Answer from the drawing. Dimensions are ordinates in mm from the lowest x, y and z of the part. A direction names the side the tool comes from. Give positions to 0.01 mm unless a question says otherwise; leave off trailing zeros. Loops run counter-clockwise (first coordinate to the right, second up) from the corner with the lowest first, then second, coordinate; pieces in that order, holes last.
Item 1: Consider line 1 along Z through (x, y) = (26, 83); line 2 along Y through (x, z) = (78.5, 28.5) (1 decimal); line 3 along Z through (x, y) = (77.5, 103). Determine where each line is inside the solid, lowest interval first.
Item 2: Section D-D, the plane x = 97 is taken. Give the vertices of the cut face in (y, z) (1 decimal).
Item 3: Section B-B, the plane y = 120 is taken. Give the vertices of the cut face in (x, z).
Item 4: A tool of negligible diameter and unlimited length cuts with its end or side. For the marked faces 1 and 2, from which of +Z, -Z, +X, -X, +Y, -Y can it reach the whole face along a straight path? Write none if from no direction.
Item 5: Section A-A, the plane x = 58.5 is taken. Give the vertices of the cut face in (y, z), and give its area (3 significant figures).
Item 6: Each of these flat-tipped pins is pushed along its axis until it touches: pin 1 Ø5 at (x, y) = (98, 26.5) entering from -Z; pin 2 Ø4 at (x, y) = (122, 122.5) entering from +Z; pin 3 Ø1.5 at (x, z) = (80.5, 45.5) entering from -Y. Where does it stop, or does it pass through?
Item 7: Section C-C, the plane z = 60.5 is taken. Give the vertices of the cut face in (x, y) (1 decimal), and give its area (3 significant figures).
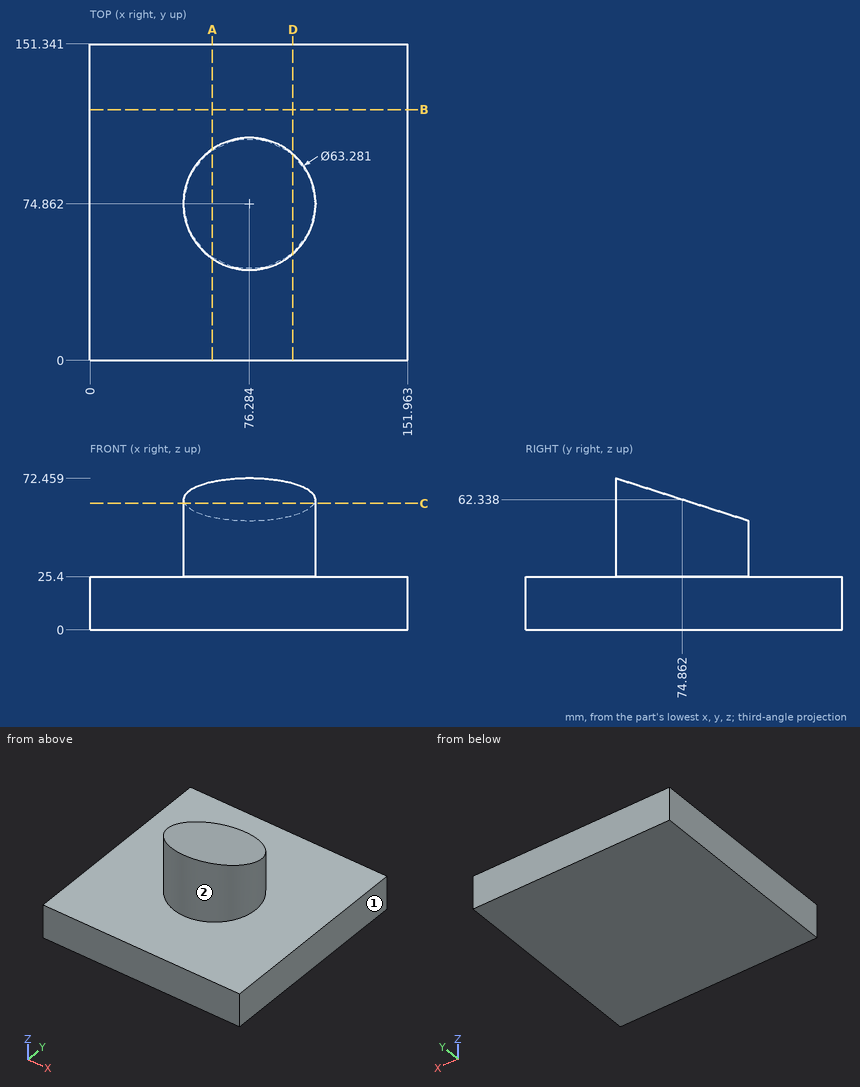
Worked answers:
1. line 1: z = 0 to 25.4
1. line 2: y = 43.3 to 106.4
1. line 3: z = 0 to 53.34
2. outline: (0, 0) - (151.3, 0) - (151.3, 25.4) - (98.8, 25.4) - (98.8, 54.7) - (50.9, 70) - (50.9, 25.4) - (0, 25.4) - close
3. outline: (0, 0) - (151.96, 0) - (151.96, 25.4) - (0, 25.4) - close
4. face 1: +Z, -Z, +X, +Y, -Y
4. face 2: +Z
5. outline: (0, 0) - (151.34, 0) - (151.34, 25.4) - (101.03, 25.4) - (101.03, 53.97) - (48.69, 70.71) - (48.69, 25.4) - (0, 25.4) - close
5. area: 5,780 mm2
6. pin 1: stops at z = 0
6. pin 2: stops at z = 25.4
6. pin 3: stops at y = 43.41
7. outline: (45.2, 80.6) arc R31.6 ccw (long way) to (107.4, 80.6) - close
7. area: 1,930 mm2
